Design review of the part shown in the three views and the two pictorial views. Dimensions are in mm from the part's minimum x, y and z. Coordinates: 2 decimals unless noted, no trailing zeros. Write each loop counter-clockwise with the first axis right and the second up, starting at its lowest first coordinate (ties: lowest second). Pieces come first, ordered by that corner, then holes. Notation, with made-up numbers: M 16,25 L 25,25 A20 ccw 25,54 Z; hole C -21,-23 d8. An arc over 180 degrees is marked long. Answer as a JSON object with one key per item and string values.
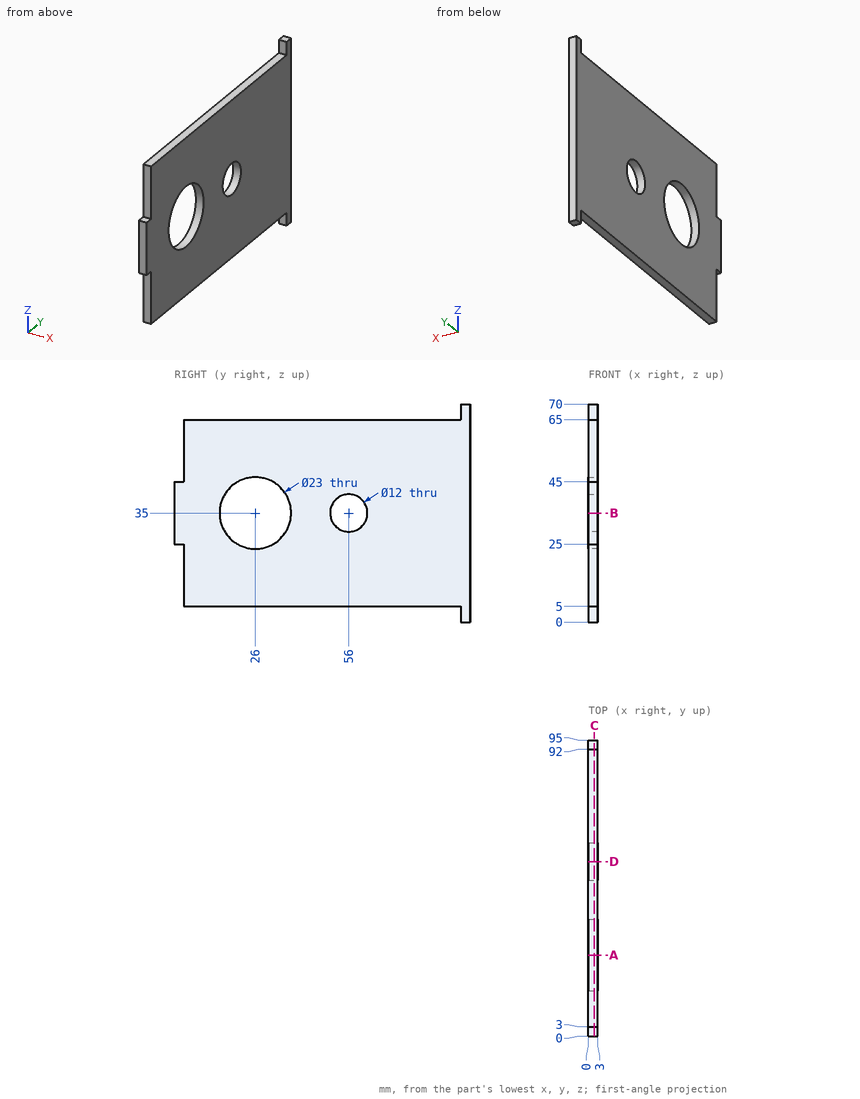
(1) For pin 1 Ø14 at (y, z) = (56, 35) entering from -X; pin 2 Ø1.5 at (x, z) = (2, 2.5) entering from -Y; pin 3 Ø0.9 at (x, y) = (2, 1) entering from -Z; pin 4 Ø1.5 at (x, y) = (1.5, 69) entering from -Z, all flat-tipped, find the tip position at first contact; note any pin that passes through.
Results list:
{"pin 1": "x = 0", "pin 2": "y = 92", "pin 3": "z = 25", "pin 4": "z = 5"}
(2) Add section B-B on z = 35. Give the boundary of the cut face in (x, y), and give its area (3 significant figures).
Results list:
{"outline": "M 0,0 L 3,0 L 3,14.5 L 0,14.5 Z; M 0,37.5 L 3,37.5 L 3,50 L 0,50 Z; M 0,62 L 3,62 L 3,95 L 0,95 Z", "area": "180 mm²"}
(3) Wall thickness on line 1 along Y through (x, z) = (1.35, 35); line 2 along Y through (x, z) = (1.75, 31); line 3 along Z through (x, y) = (2.6, 68): over which ranges is each line inside the solid? List them lowest first. Write a range as from..to.
Results list:
{"line 1": "0..14.5, 37.5..50, 62..95", "line 2": "0..15.22, 36.78..51.53, 60.47..95", "line 3": "5..65"}
(4) Add section A-A on y = 26. Give the boundary of the cut face in (x, z), and give its area (3 significant figures).
Results list:
{"outline": "M 0,5 L 3,5 L 3,23.5 L 0,23.5 Z; M 0,46.5 L 3,46.5 L 3,65 L 0,65 Z", "area": "111 mm²"}
(5) Add section D-D on y = 56. Give the boundary of the cut face in (x, z).
Results list:
{"outline": "M 0,5 L 3,5 L 3,29 L 0,29 Z; M 0,41 L 3,41 L 3,65 L 0,65 Z"}
(6) Add section C-C on x = 1.95. Give the boundary of the cut face in (y, z).
Results list:
{"outline": "M 0,25 L 3,25 L 3,5 L 92,5 L 92,0 L 95,0 L 95,70 L 92,70 L 92,65 L 3,65 L 3,45 L 0,45 Z; hole C 26,35 d23; hole C 56,35 d12"}
